For this review, take the finished solid that the model builds, in its own axes (mm). Coordinates: 2 decimals unless noted, no trailing zeros. Loops run counter-clockwise (first coordinate to the right, second up) from the corner with the lowest first, then second, coordinate; pieces in that order, holes last.
1. To check wall thickness, follow probe 1 along Y at (x, z) = (78.65, 2.6); probe 2 along Y at (x, z) = (12.65, 2.4). State the ranges of each line that lie inside material, in increasing order.
2. Clearance check with flat-ended pins moving along their axes: P1, Ø4, axis at x = 12.65, y = 54.6, coming from the +Z side; P2, Ø6.5, axis at x = 122.65, y = 54.6, coming from the -Z side. State where each tip first meets the part, or that it passes through.
3. Take a section at B-B, the plane z = 1.7. Count the separate pieces of the cut face and the enclosed holes in it, then the cut area to 3 significant figures.
4. Take a section at A-A, the plane x = 166.65. State the section outline as (y, z) points.
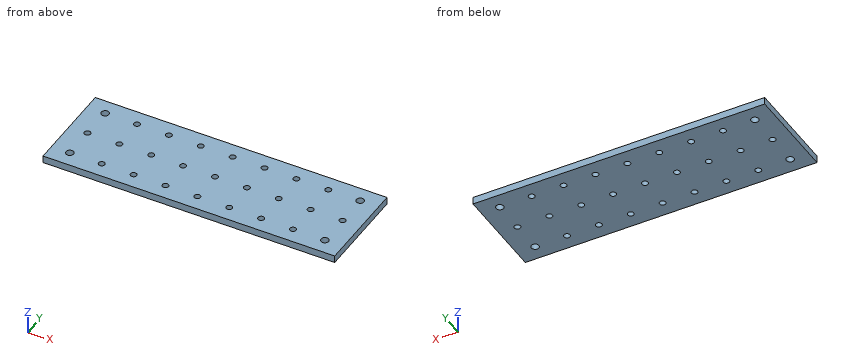
```python
from build123d import *

# Parameters (mm, degrees)
ESBO_O1_W                  = 201.3
ESBO_O1_H                  = 65.2
RESSALTO_EXTRUS_O1_DEPTH   = 5
ESBO_O2_R                  = 2.1
CORTE_EXTRUS_O1_DEPTH      = 30
ESBO_O3_R                  = 2.6
CORTE_EXTRUS_O2_DEPTH      = 28
CORTE_EXTRUS_O2_DEPTH_BACK = 22


with BuildPart() as part:
    # Esboço1 → Ressalto-extrusão1 (new body)
    with BuildSketch(Plane.XY):
        with Locations((100.65, 32.6)):
            Rectangle(ESBO_O1_W, ESBO_O1_H)
    extrude(amount=RESSALTO_EXTRUS_O1_DEPTH)

    # Esboço2 → Corte-extrusão1 (cut)
    with BuildSketch(Plane.XY):
        with Locations((100.65, 32.6)):
            Circle(ESBO_O2_R)
        with Locations((100.65, 54.6)):
            Circle(ESBO_O2_R)
        with Locations((100.65, 10.6)):
            Circle(ESBO_O2_R)
        with Locations((122.65, 32.6)):
            Circle(ESBO_O2_R)
        with Locations((122.65, 54.6)):
            Circle(ESBO_O2_R)
        with Locations((122.65, 10.6)):
            Circle(ESBO_O2_R)
        with Locations((144.65, 32.6)):
            Circle(ESBO_O2_R)
        with Locations((144.65, 54.6)):
            Circle(ESBO_O2_R)
        with Locations((144.65, 10.6)):
            Circle(ESBO_O2_R)
        with Locations((166.65, 32.6)):
            Circle(ESBO_O2_R)
        with Locations((166.65, 54.6)):
            Circle(ESBO_O2_R)
        with Locations((166.65, 10.6)):
            Circle(ESBO_O2_R)
        with Locations((188.65, 32.6)):
            Circle(ESBO_O2_R)
        with Locations((188.65, 54.6)):
            Circle(ESBO_O2_R)
        with Locations((188.65, 10.6)):
            Circle(ESBO_O2_R)
        with Locations((78.65, 32.6)):
            Circle(ESBO_O2_R)
        with Locations((78.65, 54.6)):
            Circle(ESBO_O2_R)
        with Locations((78.65, 10.6)):
            Circle(ESBO_O2_R)
        with Locations((56.65, 32.6)):
            Circle(ESBO_O2_R)
        with Locations((56.65, 54.6)):
            Circle(ESBO_O2_R)
        with Locations((56.65, 10.6)):
            Circle(ESBO_O2_R)
        with Locations((34.65, 32.6)):
            Circle(ESBO_O2_R)
        with Locations((34.65, 54.6)):
            Circle(ESBO_O2_R)
        with Locations((34.65, 10.6)):
            Circle(ESBO_O2_R)
        with Locations((12.65, 32.6)):
            Circle(ESBO_O2_R)
        with Locations((12.65, 54.6)):
            Circle(ESBO_O2_R)
        with Locations((12.65, 10.6)):
            Circle(ESBO_O2_R)
    extrude(amount=CORTE_EXTRUS_O1_DEPTH, mode=Mode.SUBTRACT)

    # Esboço3 → Corte-extrusão2 (cut, two sides)
    with BuildSketch(Plane(origin=(0, 0, 0), x_dir=(-1, 0, 0), z_dir=(0, 0, -1))) as corte_extrus_o2_sk:
        with Locations((-188.65, 54.6)):
            Circle(ESBO_O3_R)
        with Locations((-12.65, 54.6)):
            Circle(ESBO_O3_R)
        with Locations((-12.65, 10.6)):
            Circle(ESBO_O3_R)
        with Locations((-188.65, 10.6)):
            Circle(ESBO_O3_R)
    extrude(amount=CORTE_EXTRUS_O2_DEPTH, mode=Mode.SUBTRACT)
    extrude(corte_extrus_o2_sk.sketch, amount=-CORTE_EXTRUS_O2_DEPTH_BACK, mode=Mode.SUBTRACT)


solid = part.part
```
Results list:
1. probe 1: y = 0 to 8.5, 12.7 to 30.5, 34.7 to 52.5, 56.7 to 65.2
1. probe 2: y = 0 to 8, 13.2 to 30.5, 34.7 to 52, 57.2 to 65.2
2. P1: passes through
2. P2: stops at z = 0
3. separate pieces: 1
3. enclosed holes: 27
3. area: 12,700 mm2
4. outline: (0, 0) - (8.5, 0) - (8.5, 5) - (0, 5) - close; (12.7, 0) - (30.5, 0) - (30.5, 5) - (12.7, 5) - close; (34.7, 0) - (52.5, 0) - (52.5, 5) - (34.7, 5) - close; (56.7, 0) - (65.2, 0) - (65.2, 5) - (56.7, 5) - close
